Autodesk Inventor part; units mm, degrees
ref_plane "YZ Plane" through (0, 0, 0) normal (1, 0, 0) x (0, 1, 0)
ref_plane "XZ Plane" through (0, 0, 0) normal (0, 1, 0) x (-1, 0, 0)
ref_plane "XY Plane" through (0, 0, 0) normal (0, 0, 1) x (1, 0, 0)
sketch "Sketch1" plane through (0, 0, 0) normal (0, 0, 1) x (1, 0, 0)
  circle A0 centre (0, 0) radius 8
  line L0 (5.2915, -6) -> (-5.2915, -6)
  line L1 (-5.2915, -6) -> (-5.2915, 6)
  line L2 (-5.2915, 6) -> (5.2915, 6)
  line L3 (5.2915, 6) -> (5.2915, -6)
  line L4 (5.2915, -6) -> (-5.2915, 6) construction
  line L5 (-5.2915, -6) -> (5.2915, 6) construction
  point P0 (-5.2915, -6)
  point P1 (5.2915, -6)
  point P2 (5.2915, 6)
  dimension "d0" = 16
  dimension "d1" = 12
extrude "Extrusion1" add sketch "Sketch1" along normal blind 6.35 contours A0 L3 | L3 L0 L1 L2 | L1 A0
sketch "Sketch2" plane through (0, 0, 6.35) normal (0, 0, 1) x (1, 0, 0)
  arc A0 (-5.2915, 6) -> (-5.2915, -6) centre (0, 0) ccw
hole "Hole1" at (0, 0, 6.35) direction (0, 0, -1) diameter 4.134 end through all
properties part number "Print Bed Washers" material "Aluminum 6061"
Verification items for the finished model (mm, model axes). Give positions to 0.01 mm unless a question says otherwise; leave off trailing zeros. Order: outer loops, then holes, each group sorted by start corner. A loop starts at its lowest first (then second) coordinate and runs counter-clockwise, first axis right, second up. Notation, with made-up numbers: (19, 36) -> (27, 36) arc R38 ccw to (27, 75) -> close; hole circle Ø11 at (-19.5, 87.25). An arc over 180 degrees is marked (long way). Use a Markdown table: item, result.
1) Section check D-D, the plane x = -6. Record the boundary of the cut face in (y, z), then the cut area to 3 significant figures.
Results:
| item | result |
|---|---|
| outline | (-5.29, 0) -> (5.29, 0) -> (5.29, 6.35) -> (-5.29, 6.35) -> close |
| area | 67.2 mm² |
2) Material ranges on probe 1 along X at (y, z) = (0, 4.5); probe 2 along Y at (x, z) = (0, 3); probe 3 along Y at (x, z) = (0.75, 2.75), recorded low to high.
Results:
| item | result |
|---|---|
| probe 1 | -8 to -2.07, 2.07 to 8 |
| probe 2 | -6 to -2.07, 2.07 to 6 |
| probe 3 | -6 to -1.93, 1.93 to 6 |
3) Mould release check, pull along X, two halves, no side actions. Record for faces 1 (the cylindrical face through (-8, 0, 3)), 2 (the cylindrical face through (1.26, 1.64, 3.13)), 3 (the flat face through (-2, 1, 0)): pulls with the +X half, pulls with the -X half, needs draft (parallel to the pull), parting line crosses it, or undercut.
Results:
| item | result |
|---|---|
| face 1 | pulls with the -X half |
| face 2 | undercut |
| face 3 | needs draft |
4) Section check A-A, the plane x = -1.75. Record the boundary of the cut face in (y, z), then the cut area to 3 significant figures.
Results:
| item | result |
|---|---|
| outline | (-6, 0) -> (-1.1, 0) -> (-1.1, 6.35) -> (-6, 6.35) -> close; (1.1, 0) -> (6, 0) -> (6, 6.35) -> (1.1, 6.35) -> close |
| area | 62.2 mm² |
5) Section check B-B, the plane y = 0. Record the boundary of the cut face in (x, z).
Results:
| item | result |
|---|---|
| outline | (-8, 0) -> (-2.07, 0) -> (-2.07, 6.35) -> (-8, 6.35) -> close; (2.07, 0) -> (8, 0) -> (8, 6.35) -> (2.07, 6.35) -> close |
6) Section check C-C, the plane z = 4.25. Record the boundary of the cut face in (x, y).
Results:
| item | result |
|---|---|
| outline | (-5.29, -6) -> (5.29, -6) arc R8 ccw to (5.29, 6) -> (-5.29, 6) arc R8 ccw to start; hole circle Ø4.13 at (0, 0) |
